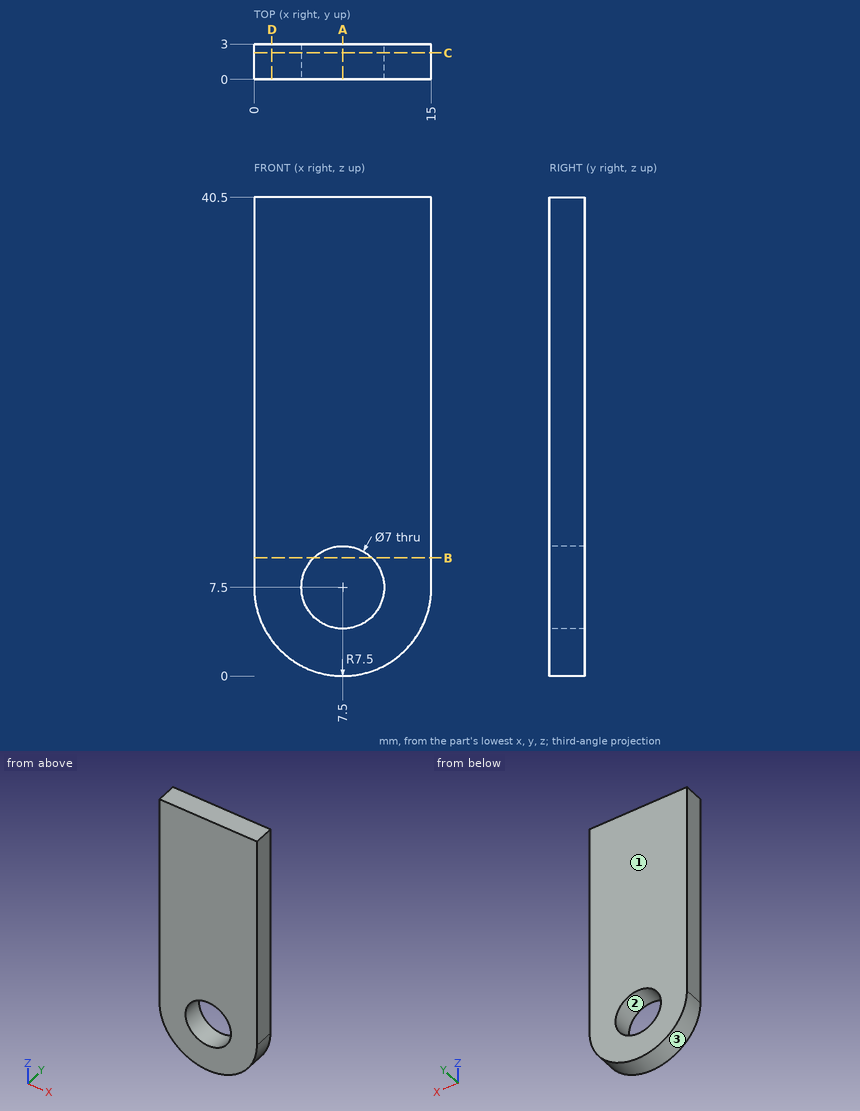
Geometry: see drawing. Coordinates: mm, zero at the bounding-box minimum. Coordinates: 2 decimals unless noted, no trailing zeros. Order: outer loops, then holes, each group sorted by start corner. A loop starts at its lowest first (then second) coordinate and runs counter-clockwise, first axis right, second up. Notation, with made-up numbers: (31.25, 13) - (77.25, 13) arc R6 cw to (77.25, 24) - close; hole circle Ø7 at (-33, 0.25). An arc over 180 degrees is marked (long way). Use one line per item in the form item = value.
1) Section B-B (z = 10). Return loops of the section in (x, y), then the cut area to 3 significant figures.
Solutions:
outline = (0, 0) - (5.05, 0) - (5.05, 3) - (0, 3) - close; (9.95, 0) - (15, 0) - (15, 3) - (9.95, 3) - close
area = 30.3 mm^2
2) Ray query, L1, parallel to Z at x = 7.75, y = 1.95; L2, parallel to X at y = 1.9, z = 7.5; L3, parallel to Z at x = 1.5, y = 2.7. Return the intervals inside material, ascending.
Solutions:
L1 = 0 to 4.01, 10.99 to 40.5
L2 = 0 to 4, 11 to 15
L3 = 3 to 40.5
3) Section C-C (y = 2.25). Return loops of the section in (x, z).
Solutions:
outline = (0, 7.5) arc R7.5 ccw to (15, 7.5) - (15, 40.5) - (0, 40.5) - close; hole circle Ø7 at (7.5, 7.5)
4) Mould query, pull axis X, two halves, no side actions, for the marked faces 1, 2 and 3. Classes: +X half, -X half, draft (parallel to the pull), parting line (faces both ways), or undercut.
Solutions:
face_1 = draft
face_2 = undercut
face_3 = parting line
5) Section A-A (x = 7.5). Return loops of the section in (y, z).
Solutions:
outline = (0, 0) - (3, 0) - (3, 4) - (0, 4) - close; (0, 11) - (3, 11) - (3, 40.5) - (0, 40.5) - close
6) Section D-D (x = 1.5). Return loops of the section in (y, z).
Solutions:
outline = (0, 3) - (3, 3) - (3, 40.5) - (0, 40.5) - close
